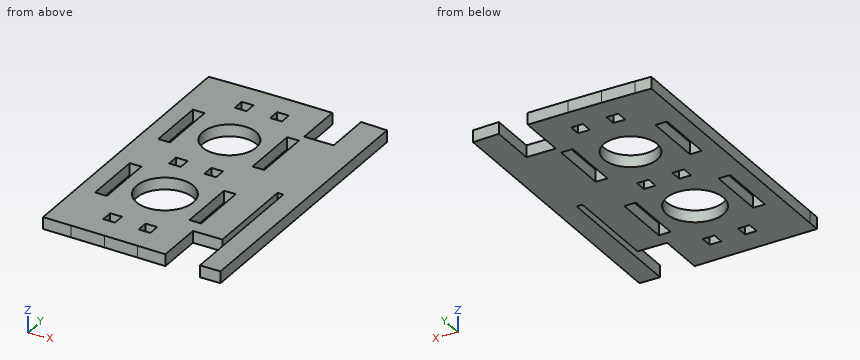
from build123d import *

# Parameters (mm, degrees)
MODEL_R         = 4.534410691
MODEL_R_2       = 4.826928656
MODEL_W         = 2
MODEL_H         = 10
MODEL_H_2       = 2
EXTRUDE_1_DEPTH = 2


with BuildPart() as part:
    # Model → 凸台-拉伸1 (new body)
    with BuildSketch(Plane.XY):
        Polygon((883.637204973, 587.330530622), (886.356553012, 587.393355998), (892.052378601, 587.452861056), (897.748434881, 587.438305688), (904.608822678, 587.348603606), (904.608822678, 579.211202345), (909.608822678, 579.211202345), (909.608822678, 580.211202345), (909.608822678, 587.161390594), (914.108822678, 586.966954635), (914.108822678, 579.859457913), (914.108822678, 538.869007346), (910.608822678, 538.869007346), (910.608822678, 562.993038329), (909.608822678, 562.993038329), (909.608822678, 547.086608467), (904.608822678, 547.086608467), (904.608822678, 539.117249216), (899.835523647, 539.223453365), (894.140406006, 539.331138315), (888.444075417, 539.420753158), (883.636881049, 539.481070293), (883.637204973, 541.525037946), align=None)
        with Locations((895.661921161, 572.865848158)):
            Circle(MODEL_R, mode=Mode.SUBTRACT)
        with Locations((895.579584436, 554.362843803)):
            Circle(MODEL_R_2, mode=Mode.SUBTRACT)
        with Locations((887.540358452, 554.584784532)):
            Rectangle(MODEL_W, MODEL_H, mode=Mode.SUBTRACT)
        with Locations((887.540358452, 572.817915241)):
            Rectangle(MODEL_W, MODEL_H, mode=Mode.SUBTRACT)
        with Locations((903.540358452, 572.817915241)):
            Rectangle(MODEL_W, MODEL_H, mode=Mode.SUBTRACT)
        with Locations((903.540358452, 554.584784532)):
            Rectangle(MODEL_W, MODEL_H, mode=Mode.SUBTRACT)
        with Locations((898.540358452, 544.428876798)):
            Rectangle(MODEL_W, MODEL_H_2, mode=Mode.SUBTRACT)
        with Locations((892.540358452, 544.428876798)):
            Rectangle(MODEL_W, MODEL_H_2, mode=Mode.SUBTRACT)
        with Locations((898.540358452, 563.428876798)):
            Rectangle(MODEL_W, MODEL_H_2, mode=Mode.SUBTRACT)
        with Locations((892.540358452, 563.428876798)):
            Rectangle(MODEL_W, MODEL_H_2, mode=Mode.SUBTRACT)
        with Locations((898.540358452, 582.428876798)):
            Rectangle(MODEL_W, MODEL_H_2, mode=Mode.SUBTRACT)
        with Locations((892.540358452, 582.428876798)):
            Rectangle(MODEL_W, MODEL_H_2, mode=Mode.SUBTRACT)
    extrude(amount=EXTRUDE_1_DEPTH)


solid = part.part
Can you work these out from the model? Positions are in its coordinate system, mm. Give positions to 0.01 mm unless a question says otherwise; leave off trailing zeros. Loops run counter-clockwise (first coordinate to the right, second up) from the corner with the lowest first, then second, coordinate; pieces in that order, holes last. Notation, with made-up numbers: M -35.75,-1 L 20.25,-1 A22 ccw 20.25,24 Z; hole C 82,0.5 d3. An arc over 180 degrees is marked long. One line per item, written item: value. Start each with the question number.
1) I'm going to push flat-ended pins straight in: pin 1 (1 mm diameter, centred on x = 892.5, z = 1.5, fed in from -Y); pin 2 (1 mm diameter, centred on x = 890, z = 1.5, fed in from -Y); pin 3 (1 mm diameter, centred on x = 898, z = 1, fed in from +Y). Where does each tip first touch, or does it pass through?
2) If we section it at A-A, the plane y = 546.5: Write out the boundary of the cut face in (x, z).
3) If we section it at C-C, the plane y = 571: Write out the boundary of the cut face in (x, z), and give its area (3 significant figures).
4) If we section it at D-D, the plane y = 580: Write out the boundary of the cut face in (x, z), and give its area (3 significant figures).
5) If we section it at B-B, the plane x = 895: Write out the boundary of the cut face in (y, z), and give its area (3 significant figures).
6) If I drill on line 1 (X direction, y = 545, z = 0.25); line 2 (X direction, y = 568, z = 0.15); line 3 (X direction, y = 558, z = 1), over which ranges is the centre line in solid material (lowest first)? Write a range as [from, to].
Completed:
1. pin 1: stops at y = 539.35
1. pin 2: stops at y = 539.39
1. pin 3: stops at y = 587.44
2. outline: M 883.64,0 L 904.61,0 L 904.61,2 L 883.64,2 Z; M 910.61,0 L 914.11,0 L 914.11,2 L 910.61,2 Z
3. outline: M 883.64,0 L 886.54,0 L 886.54,2 L 883.64,2 Z; M 888.54,0 L 891.53,0 L 891.53,2 L 888.54,2 Z; M 899.79,0 L 902.54,0 L 902.54,2 L 899.79,2 Z; M 904.54,0 L 914.11,0 L 914.11,2 L 904.54,2 Z
3. area: 36.4 mm^2
4. outline: M 883.64,0 L 904.61,0 L 904.61,2 L 883.64,2 Z; M 909.61,0 L 914.11,0 L 914.11,2 L 909.61,2 Z
4. area: 50.9 mm^2
5. outline: M 539.31,0 L 549.57,0 L 549.57,2 L 539.31,2 Z; M 559.15,0 L 568.38,0 L 568.38,2 L 559.15,2 Z; M 577.35,0 L 587.45,0 L 587.45,2 L 577.35,2 Z
5. area: 59.1 mm^2
6. line 1: x = [883.64, 891.54], [893.54, 897.54], [899.54, 904.61], [910.61, 914.11]
6. line 2: x = [883.64, 886.54], [888.54, 902.54], [904.54, 914.11]
6. line 3: x = [883.64, 886.54], [888.54, 892.41], [898.75, 902.54], [904.54, 909.61], [910.61, 914.11]
